Source: CAD feature listing. Evaluate the final solid. Frame: model axes, mm. A direction names the side the tool comes from. Give positions to 0.01 mm unless a question says otherwise; leave off trailing zeros. Write each loop counter-clockwise with the first axis right and the second up, starting at its lowest first coordinate (ties: lowest second). Pieces come first, ordered by that corner, then holes. Notation, with made-up numbers: (57.5, 73) -> (88.5, 73) arc R15 cw to (88.5, 80) -> close; hole circle Ø5 at (-26.5, 76). An arc over 180 degrees is marked (long way). Write item = value, one per line.
from build123d import *

# Parameters (mm, degrees)
F0_R     = 44.45
F1_DEPTH = 29.21
F2_SIZE  = 3.175
F3_R     = 13.462
F4_DEPTH = 38.1
F5_R     = 10.922
F6_DEPTH = 25.4


with BuildPart() as f1:
    # F0 (on Top) → F1 (new body)
    with BuildSketch(Plane.XY):
        Circle(F0_R)
    extrude(amount=F1_DEPTH)

    # F2
    f2_edges = [f1.edges().sort_by_distance(p)[0] for p in [
        (-44.45, 0, 0),
    ]]
    chamfer(f2_edges, length=F2_SIZE)

    # F3 (on face) → F4 (join)
    with BuildSketch(Plane(origin=(0, 0, 0), x_dir=(1, 0, 0), z_dir=(0, 0, -1))):
        Circle(F3_R)
    extrude(amount=F4_DEPTH)

    # F5 (on face) → F6 (join)
    with BuildSketch(Plane(origin=(0, 0, -38.1), x_dir=(1, 0, 0), z_dir=(0, 0, -1))):
        Circle(F5_R)
    extrude(amount=F6_DEPTH)


solid = f1.part
1) Cut plane D-D (z = 21.5). Return the cut outline in (x, y).
Computed:
outline = circle Ø88.9 at (0, 0)
2) Cut plane A-A (y = 0). Return the cut outline in (x, z) (3 decimals), then the cut area to 3 significant figures.
Computed:
outline = (-44.45, 3.175) -> (-41.275, 0) -> (-13.462, 0) -> (-13.462, -38.1) -> (-10.922, -38.1) -> (-10.922, -63.5) -> (10.922, -63.5) -> (10.922, -38.1) -> (13.462, -38.1) -> (13.462, 0) -> (41.275, 0) -> (44.45, 3.175) -> (44.45, 29.21) -> (-44.45, 29.21) -> close
area = 4,170 mm²
3) Contact query for flat-ended pins moving along their axis: pin 1 (8 mm diameter, centred on x = -17.5, y = 34, fed in from -Z); pin 2 (2 mm diameter, centred on x = 12, y = -4, fed in from -Z); pin 3 (1.5 mm diameter, centred on x = 8, z = -41.5, fed in from -Y). Output: stop coordinate, or through.
Computed:
pin_1 = 0
pin_2 = -38.1
pin_3 = -8.17
4) Cut plane C-C (z = -53). Return the cut outline in (x, y).
Computed:
outline = circle Ø21.84 at (0, 0)
5) Material intervals for L1, parallel to Z at x = 25, y = -30; L2, parallel to X at y = -32.5, z = 16; L3, parallel to Y at x = -18.5, z = 5.5, sorted ascending.
Computed:
L1 = 0 to 29.21
L2 = -30.32 to 30.32
L3 = -40.42 to 40.42
6) Access query for faces 1 (the cylindrical face through (10.418, -3.281, -50.622)), 2 (the flat face through (0, 0, -63.5)). Directions: +Z, -Z, +X, -X, +Y, -Y. A direction counts if a zero-diameter tool reaches every point of the face in a straight line with its end or side. Return the directions, or none.
Computed:
face_1 = -Z
face_2 = -Z, +X, -X, +Y, -Y
